CAD build for the part. Positions are in the model's coordinates, mm. A direction names the side the tool comes from. Round coordinates to 2 decimals unless told otherwise and drop trailing zeros. Loops run counter-clockwise (first coordinate to the right, second up) from the corner with the lowest first, then second, coordinate; pieces in that order, holes last. Notation, with made-up numbers: (23.25, -5.75) - (71.25, -5.75) arc R25 cw to (71.25, 8.25) - close; hole circle Ø4 at (83.5, 51.5). An arc over 180 degrees is marked (long way). One line per question, with ' | ' between items.
```python
from build123d import *

# Parameters (mm, degrees)
CSK_FOR_M3_HEX_SOCKET_COUNTERSUNK_HE_2_COUNT = 2
CSK_FOR_M3_HEX_SOCKET_COUNTERSUNK_HE_2_PITCH = 30


with BuildPart() as part:
    # Sketch1 → Revolve1 (revolve)
    with BuildSketch(Plane(origin=(0, 0, 0), x_dir=(1, 0, 0), z_dir=(0, 1, 0))):
        Polygon((-1.5, 21), (1.5, 21), (1.5, 11), (2.5, 11), (2.5, 9.5), (-1.5, 9.5), align=None)
    revolve(axis=Axis((88.99, 0, 0), (-1, 0, 0)))

    # Sketch3 → CSK for M3 Hex Socket Countersunk Head Screw1 (revolve, cut)
    with BuildSketch(Plane(origin=(-1.5, 0, 15), x_dir=(0, 0, 1), z_dir=(0, 1, 0))):
        Polygon((0, 0), (0, 3), (1.7, 3), (1.7, 1.77), (3.47, 0), align=None)
    csk_for_m3_hex_socket_countersunk_head_s = revolve(axis=Axis((-7.85, 0, 15), (1, 0, 0)), mode=Mode.SUBTRACT)

    # CSK for M3 Hex Socket Countersunk He 2: CSK for M3 Hex Socket Countersunk Head Screw1 ×2
    with Locations(*[(0, 0, -i * CSK_FOR_M3_HEX_SOCKET_COUNTERSUNK_HE_2_PITCH) for i in range(1, CSK_FOR_M3_HEX_SOCKET_COUNTERSUNK_HE_2_COUNT)]):
        add(csk_for_m3_hex_socket_countersunk_head_s, mode=Mode.SUBTRACT)


solid = part.part
```
(1) Cut at B-B, the plane y = 0. Write the cut outline in (x, z), then the cut area to 3 significant figures.
Results found:
outline: (-1.5, -21) - (1.5, -21) - (1.5, -16.7) - (0.27, -16.7) - (-1.5, -18.47) - close; (-1.5, -11.53) - (0.27, -13.3) - (1.5, -13.3) - (1.5, -11) - (2.5, -11) - (2.5, -9.5) - (-1.5, -9.5) - close; (-1.5, 9.5) - (2.5, 9.5) - (2.5, 11) - (1.5, 11) - (1.5, 13.3) - (0.27, 13.3) - (-1.5, 11.53) - close; (-1.5, 18.47) - (0.27, 16.7) - (1.5, 16.7) - (1.5, 21) - (-1.5, 21) - close | area: 45.3 mm²
(2) Tool access for faces 1 (the face through (0.159, -1.795, 14.764)), 2 (the face through (2.01, 10.74, 2.38)): list every direction of +Z, -Z, +X, -X, +Y, -Y with a clear straight run to the whole face (end or side of a thin tool).
Results found:
face 1: -X | face 2: +X
(3) Cut at C-C, the plane x = -0.9. Write the cut outline in (y, z).
Results found:
outline: circle Ø42 at (0, 0); hole circle Ø19 at (0, 0); hole circle Ø5.74 at (0, -15); hole circle Ø5.74 at (0, 15)
(4) Cut at A-A, the plane z = 0. Write the cut outline in (x, y), then the cut area to 3 significant figures.
Results found:
outline: (-1.5, -21) - (1.5, -21) - (1.5, -11) - (2.5, -11) - (2.5, -9.5) - (-1.5, -9.5) - close; (-1.5, 9.5) - (2.5, 9.5) - (2.5, 11) - (1.5, 11) - (1.5, 21) - (-1.5, 21) - close | area: 72.0 mm²
(5) Two-plate mould, pull along Y, no slides. Class faces 3 (the face through (0.02, -6.31, -20.03)), 4 (the face through (-1.5, 0, -10)), 5 (the face through (0.88, -0.51, -13.38)): released by +Y, released by -Y, zero draft, split by the parting line, or undercut.
Results found:
face 3: split by the parting line | face 4: zero draft | face 5: undercut
(6) Cut at D-D, the plane z = 5.5. Write the cut outline in (x, y).
Results found:
outline: (-1.5, -20.27) - (1.5, -20.27) - (1.5, -9.53) - (2.5, -9.53) - (2.5, -7.75) - (-1.5, -7.75) - close; (-1.5, 7.75) - (2.5, 7.75) - (2.5, 9.53) - (1.5, 9.53) - (1.5, 20.27) - (-1.5, 20.27) - close
(7) Probe L1, parallel to Z at x = 1, y = 0; L2, parallel to Z at x = -0.9, y = -0.5; L3, parallel to Z at x = 0.4, y = 2. List the from-to ranges inside material, lowest first.
Results found:
L1: z = -21 to -16.7, -13.3 to -9.5, 9.5 to 13.3, 16.7 to 21 | L2: z = -20.99 to -17.83, -12.17 to -9.49, 9.49 to 12.17, 17.83 to 20.99 | L3: z = -20.9 to -9.29, 9.29 to 20.9
(8) Drop flat-ended pins along their axis: P1, Ø1.5, axis at x = 0.5, z = -13.5, coming from the -Y side; P2, Ø1.5, axis at x = -1, y = 14.5, coming from the -Z side; P3, Ø1.5, axis at x = 0.5, y = -13.5, coming from the +Z side. Give the stop position or say it passes through.
Results found:
P1: stops at y = -16.69 | P2: stops at z = -15.87 | P3: stops at z = 16.69
